Check sheet for the modelled part. Datum: model origin and axes. Units: mm. Face numbers are marked on the shaded views. A direction names the side the tool comes from. Round coordinates to 2 decimals unless told otherwise and drop trailing zeros. Order: outer loops, then holes, each group sorted by start corner. A loop starts at its lowest first (then second) coordinate and runs counter-clockwise, first axis right, second up.
Q1. Set-up check for the marked faces 1 and 2: record each of +Z, -Z, +X, -X, +Y, -Y from which the full face is reachable in a straight line by a thin tool's end or side.
Q2. Cross-section at C-C on x = -6. Record the cut outline in (y, z).
Q3. Cross-section at B-B on z = 0. Record the cut outline in (x, y), then the cut area to 3 significant figures.
Q4. Scan lines: probe 1 along Y at (x, z) = (-4.5, 5.75); probe 2 along Z at (x, y) = (5, 15.5); probe 3 along Z at (x, y) = (7, 5). Record each from-to range of solid material in increasing order.
Q5. Cross-section at A-A on y = 16. Record the cut outline in (x, z), then the cut area to 3 significant figures.
Q6. Depth check by flat-ended pin: P1, Ø1, axis at x = 6.5, z = -5.5, coming from the -Y side. Enter the tip coordinate at first touch or a pass-through.
Q7. Mould release check, pull along Z, two halves, no side actions. Record for the marked faces 3, 4 and 5: +Z half, -Z half, draft (parallel to the pull), parting line (faces both ways), or undercut.
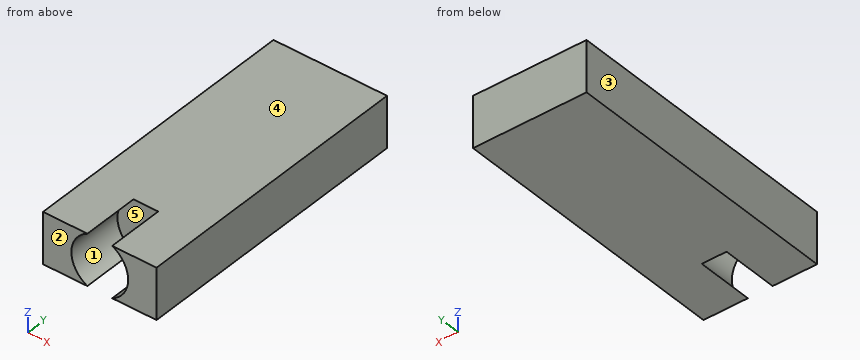
from build123d import *

# Parameters (mm, degrees)
SKETCH1_W           = 40
SKETCH1_H           = 18
BOSS_EXTRUDE1_DEPTH = 100
SKETCH3_R           = 10
SKETCH3_R_2         = 5
CUT_EXTRUDE2_DEPTH  = 20


with BuildPart() as part:
    # Sketch1 → Boss-Extrude1 (new body)
    with BuildSketch(Plane(origin=(0, 0, 0), x_dir=(1, 0, 0), z_dir=(0, 1, 0))):
        Rectangle(SKETCH1_W, SKETCH1_H)
    extrude(amount=BOSS_EXTRUDE1_DEPTH)

    # Sketch3 → Cut-Extrude2 (cut)
    with BuildSketch(Plane.XZ):
        Circle(SKETCH3_R)
        with Locations((0, 22)):
            Circle(SKETCH3_R_2)
        with Locations((0, -22)):
            Circle(SKETCH3_R_2)
    extrude(amount=-CUT_EXTRUDE2_DEPTH, mode=Mode.SUBTRACT)


solid = part.part
Results found:
1. face 1: -Y
1. face 2: +Z, -Z, +X, -X, -Y
2. outline: (0, -9) - (100, -9) - (100, 9) - (0, 9) - (0, 8) - (20, 8) - (20, -8) - (0, -8) - close
3. outline: (-20, 0) - (-10, 0) - (-10, 20) - (10, 20) - (10, 0) - (20, 0) - (20, 100) - (-20, 100) - close
3. area: 3,600 mm2
4. probe 1: y = 20 to 100
4. probe 2: z = -9 to -8.66, 8.66 to 9
4. probe 3: z = -9 to -7.14, 7.14 to 9
5. outline: (-20, -9) - (-4.36, -9) arc R10 cw to (-4.36, 9) - (-20, 9) - close; (4.36, -9) - (20, -9) - (20, 9) - (4.36, 9) arc R10 cw to start
5. area: 418 mm2
6. P1: stops at y = 20
7. face 3: draft
7. face 4: +Z half
7. face 5: undercut
